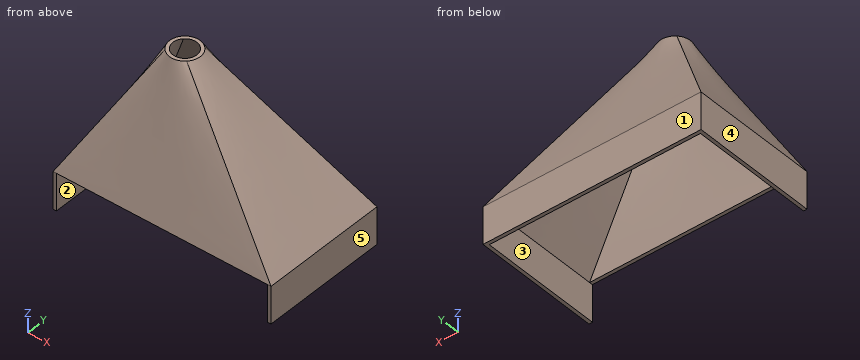
```python
from build123d import *

# Parameters (mm, degrees)
SKETCH_1_W          = 129.2
SKETCH_1_H          = 75
SKETCH_1_W_2        = 125.2
SKETCH_1_H_2        = 71
EXTRUDE_1_DEPTH     = 22
SKETCH_11_W         = 125.2
SKETCH_11_H         = 22
CUT_EXTRUDE_1_DEPTH = 10


with BuildPart() as part:
    # 草图1 → 凸台-拉伸1 (new body)
    with BuildSketch(Plane.XY):
        Rectangle(SKETCH_1_W, SKETCH_1_H)
        Rectangle(SKETCH_1_W_2, SKETCH_1_H_2, mode=Mode.SUBTRACT)
    extrude(amount=EXTRUDE_1_DEPTH)

    # 草图2 → 放样1 section 0
    with BuildSketch(Plane.XY.offset(22)):
        with BuildLine():
            Line((-64.6, 37.5), (-62.6, 35.5))
            Line((-62.6, 35.5), (62.6, 35.5))
            Line((62.6, 35.5), (64.6, 37.5))
            Line((64.6, 37.5), (-64.6, 37.5))
        make_face()
    # 草图6 for 放样1 → 放样1 section 1
    with BuildSketch(Plane.XY.offset(96)):
        with BuildLine():
            Line((-22.020458146, 4.020458146), (-23.434671709, 5.434671709))
            # circular arc as an exact rational Bezier (weights 1, cos(half-angle), 1)
            Bezier((-23.434671709, 5.434671709), (-17, 11.869343418), (-10.565328291, 5.434671709), weights=[1, 0.707106781, 1])
            Line((-10.565328291, 5.434671709), (-11.979541854, 4.020458146))
            Bezier((-11.979541854, 4.020458146), (-17, 9.040916293), (-22.020458146, 4.020458146), weights=[1, 0.707106781, 1])
        make_face()
    loft()

    # 草图3 → 放样2 section 0
    with BuildSketch(Plane.XY.offset(22)):
        with BuildLine():
            Line((-62.6, 35.5), (-64.6, 37.5))
            Line((-64.6, 37.5), (-64.6, -37.5))
            Line((-64.6, -37.5), (-62.6, -35.5))
            Line((-62.6, -35.5), (-62.6, 35.5))
        make_face()
    # 草图7 for 放样2 → 放样2 section 1
    with BuildSketch(Plane.XY.offset(96)):
        with BuildLine():
            Line((-22.020458146, 4.020458146), (-23.434671709, 5.434671709))
            Bezier((-23.434671709, 5.434671709), (-29.869343418, -1), (-23.434671709, -7.434671709), weights=[1, 0.707106781, 1])
            Line((-23.434671709, -7.434671709), (-22.020458146, -6.020458146))
            Bezier((-22.020458146, -6.020458146), (-27.040916293, -1), (-22.020458146, 4.020458146), weights=[1, 0.707106781, 1])
        make_face()
    loft()

    # 草图4 → 放样3 section 0
    with BuildSketch(Plane.XY.offset(22)):
        with BuildLine():
            Line((-62.6, -35.5), (-64.6, -37.5))
            Line((-64.6, -37.5), (64.6, -37.5))
            Line((64.6, -37.5), (62.6, -35.5))
            Line((62.6, -35.5), (-62.6, -35.5))
        make_face()
    # 草图8 for 放样3 → 放样3 section 1
    with BuildSketch(Plane.XY.offset(96)):
        with BuildLine():
            Line((-22.020458146, -6.020458146), (-23.434671709, -7.434671709))
            Bezier((-23.434671709, -7.434671709), (-17, -13.869343418), (-10.565328291, -7.434671709), weights=[1, 0.707106781, 1])
            Line((-10.565328291, -7.434671709), (-11.979541854, -6.020458146))
            Bezier((-11.979541854, -6.020458146), (-17, -11.040916293), (-22.020458146, -6.020458146), weights=[1, 0.707106781, 1])
        make_face()
    loft()

    # 草图5 → 放样4 section 0
    with BuildSketch(Plane.XY.offset(22)):
        with BuildLine():
            Line((64.6, 37.5), (62.6, 35.5))
            Line((62.6, 35.5), (62.6, -35.5))
            Line((62.6, -35.5), (64.6, -37.5))
            Line((64.6, -37.5), (64.6, 37.5))
        make_face()
    # 草图9 for 放样4 → 放样4 section 1
    with BuildSketch(Plane.XY.offset(96)):
        with BuildLine():
            Line((-10.565328291, 5.434671709), (-11.979541854, 4.020458146))
            Bezier((-11.979541854, 4.020458146), (-6.959083707, -1), (-11.979541854, -6.020458146), weights=[1, 0.707106781, 1])
            Line((-11.979541854, -6.020458146), (-10.565328291, -7.434671709))
            Bezier((-10.565328291, -7.434671709), (-4.130656582, -1), (-10.565328291, 5.434671709), weights=[1, 0.707106781, 1])
        make_face()
    loft()

    # 草图11 → 切除-拉伸1 (cut)
    with BuildSketch(Plane(origin=(0, -35.5, 0), x_dir=(1, 0, 0), z_dir=(0, 1, 0))):
        with Locations((0, -11)):
            Rectangle(SKETCH_11_W, SKETCH_11_H)
    extrude(amount=-CUT_EXTRUDE_1_DEPTH, mode=Mode.SUBTRACT)


solid = part.part
```
Could you check a few things on this model? Use its own coordinates, in mm. Face numbers are marked on the shaded views. A direction names the side the tool comes from. Round coordinates to 2 decimals unless told otherwise and drop trailing zeros. Put each result on its own line as item: value.
Q1. I need wall thicknesses on probe 1 along X at (y, z) = (-8, 12); probe 2 along Y at (x, z) = (-26, 48.5); probe 3 along X at (y, z) = (-18, 46). Which ranges of each line are inside material? Lowest first, please.
Check result:
probe 1: -64.6 to -62.6, 62.6 to 64.6
probe 2: -27.47 to -25.5, 24.78 to 26.75
probe 3: -51.73 to -49.77, 38.74 to 40.7
Q2. Thinking about a two-plate mould opening in X: for the marked faces 3, 4 and 5, which applies, released by +X, released by -X, zero draft, split by the parting line, or undercut?
Check result:
face 3: undercut
face 4: released by -X
face 5: released by +X
Q3. On a 3-axis mill with a long thin cutter (end or side, diameter ignored), from which of +Z, -Z, +X, -X, +Y, -Y can I reach the whole of each face in a straight line? I mean the marked faces 1 and 2. Say none if no direction works.
Check result:
face 1: +Z, -Z, +X, -X, +Y
face 2: -Z, -Y
Q4. For pin 1 (5 mm diameter, centred on x = 6, z = 76.5, fed in from +Y); pin 2 (17.5 mm diameter, centred on x = 28.5, z = 6.5, fed in from -Y); pin 3 (2 mm diameter, centred on x = 29.5, y = -29, fed in from +Z), each with a flat end and sliding along its axis, tell me the tip position at first contact or that it passes through.
Check result:
pin 1: y = 15.76
pin 2: y = 35.5
pin 3: z = 46.19
